```python
from build123d import *

# Parameters (mm, degrees)
SKETCH1_R           = 3.15
SKETCH1_R_2         = 34
BOSS_EXTRUDE2_DEPTH = 5
FILLET1_R           = 5
SKETCH2_R           = 6
CUT_EXTRUDE1_DEPTH  = 262.252751182


with BuildPart() as part:
    # Sketch1 → Boss-Extrude2 (new body)
    with BuildSketch(Plane.XY):
        Polygon((0, 0), (-44, 0), (-82, 70.398863627), (-82, 191.598863627), (-31.959298408, 248), (31.959298408, 248), (82, 191.598863627), (82, 70.398863627), (44, 0), align=None)
        with Locations((-31.449578633, 232)):
            Circle(SKETCH1_R, mode=Mode.SUBTRACT)
        with Locations((-24, 16)):
            Circle(SKETCH1_R, mode=Mode.SUBTRACT)
        with Locations((-54, 150.398863627)):
            Circle(SKETCH1_R, mode=Mode.SUBTRACT)
        with Locations(Location((24, 16, 0), (0, 0, 180))):
            Circle(SKETCH1_R, mode=Mode.SUBTRACT)
        with Locations(Location((31.449578633, 232, 0), (0, 0, 180))):
            Circle(SKETCH1_R, mode=Mode.SUBTRACT)
        with Locations(Location((54, 150.398863627, 0), (0, 0, 180))):
            Circle(SKETCH1_R, mode=Mode.SUBTRACT)
        with Locations((30, 70.398863627)):
            Circle(SKETCH1_R_2, mode=Mode.SUBTRACT)
        with BuildLine():
            Line((-37.93380879, 156.398863627), (37.93380879, 156.398863627))
            ThreePointArc((37.93380879, 156.398863627), (43.130728491, 163.664663146), (51.276643519, 167.331253579))
            ThreePointArc((51.276643519, 167.331253579), (0, 204.398863627), (-51.276643519, 167.331253579))
            ThreePointArc((-51.276643519, 167.331253579), (-43.130728491, 163.664663146), (-37.93380879, 156.398863627))
        make_face(mode=Mode.SUBTRACT)
        with BuildLine():
            Line((-51.276643519, 133.466473676), (-51.276643519, 70.398863627))
            ThreePointArc((-51.276643519, 70.398863627), (-34.638321759, 53.760541868), (-18, 70.398863627))
            ThreePointArc((-18, 70.398863627), (2.532150776, 109.762771703), (46.563219124, 115.450609123))
            ThreePointArc((46.563219124, 115.450609123), (58.841139814, 121.862892104), (51.276643519, 133.466473676))
            ThreePointArc((51.276643519, 133.466473676), (43.130728491, 137.133064108), (37.93380879, 144.398863627))
            Line((37.93380879, 144.398863627), (-37.93380879, 144.398863627))
            ThreePointArc((-37.93380879, 144.398863627), (-43.130728491, 137.133064108), (-51.276643519, 133.466473676))
        make_face(mode=Mode.SUBTRACT)
    extrude(amount=BOSS_EXTRUDE2_DEPTH)

    # Fillet1
    fillet1_edges = [part.edges().sort_by_distance(p)[0] for p in [
        (-44, 0, 2.5),
        (-82, 70.398863627, 2.5),
        (-82, 191.598863627, 2.5),
        (-31.959298408, 248, 2.5),
        (31.959298408, 248, 2.5),
        (82, 191.598863627, 2.5),
        (82, 70.398863627, 2.5),
        (44, 0, 2.5),
    ]]
    fillet(fillet1_edges, radius=FILLET1_R)

    # Sketch2 → Cut-Extrude1 (cut, through all)
    with BuildSketch(Plane(origin=(0, 0, 0), x_dir=(-1, 0, 0), z_dir=(0, 0, -1))):
        with Locations((24, 16)):
            Circle(SKETCH2_R)
        with Locations((-24, 16)):
            Circle(SKETCH2_R)
    extrude(amount=-CUT_EXTRUDE1_DEPTH, mode=Mode.SUBTRACT)


solid = part.part
```
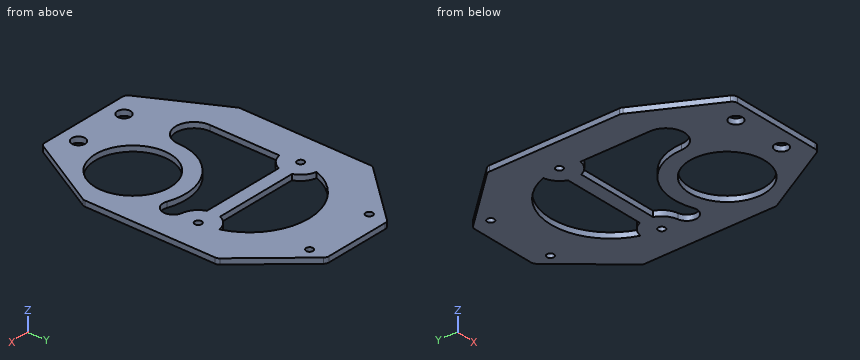
Check sheet for the modelled part. Datum: model origin and axes. Units: mm. Coordinates: 2 decimals unless noted, no trailing zeros. Loops run counter-clockwise (first coordinate to the right, second up) from the corner with the lowest first, then second, coordinate; pieces in that order, holes last.
1) Sectioned sample at D-D (y = 50). Record the boundary of the cut face in (x, z).
2) Sectioned sample at B-B (x = -24). Record the boundary of the cut face in (y, z), and give its area (3 significant figures).
3) Sectioned sample at C-C (x = -54). Record the boundary of the cut face in (y, z).
4) Sectioned sample at A-A (y = 16). Record the boundary of the cut face in (x, z).
5) Gauge pin test, flat end, axial feed: pin 1 (10 mm diameter, centred on x = -61.5, y = 180, fed in from -Z). Record the tip position at first contact, or that the pin passes through.
6) Material ranges on probe 1 along Y at (x, z) = (16, 4.15) (3 decimals); probe 2 along X at (y, z) = (232, 2.25); probe 3 along X at (y, z) = (11, 0.55), recorded low to high.
Check sheet entries:
1. outline: (-70.99, 0) - (2.8, 0) - (2.8, 5) - (-70.99, 5) - close; (57.2, 0) - (70.99, 0) - (70.99, 5) - (57.2, 5) - close
2. outline: (0, 0) - (10, 0) - (10, 5) - (0, 5) - close; (22, 0) - (57.61, 0) - (57.61, 5) - (22, 5) - close; (144.4, 0) - (156.4, 0) - (156.4, 5) - (144.4, 5) - close; (198.77, 0) - (248, 0) - (248, 5) - (198.77, 5) - close
2. area: 534 mm2
3. outline: (18.53, 0) - (147.25, 0) - (147.25, 5) - (18.53, 5) - close; (153.55, 0) - (223.16, 0) - (223.16, 5) - (153.55, 5) - close
4. outline: (-52.64, 0) - (-30, 0) - (-30, 5) - (-52.64, 5) - close; (-18, 0) - (18, 0) - (18, 5) - (-18, 5) - close; (30, 0) - (52.64, 0) - (52.64, 5) - (30, 5) - close
5. pin 1: stops at z = 0
6. probe 1: y = 0 to 39.415, 101.383 to 116.312, 144.399 to 156.399, 201.974 to 248
6. probe 2: x = -46.15 to -34.6, -28.3 to 28.3, 34.6 to 46.15
6. probe 3: x = -49.94 to -27.32, -20.68 to 20.68, 27.32 to 49.94
